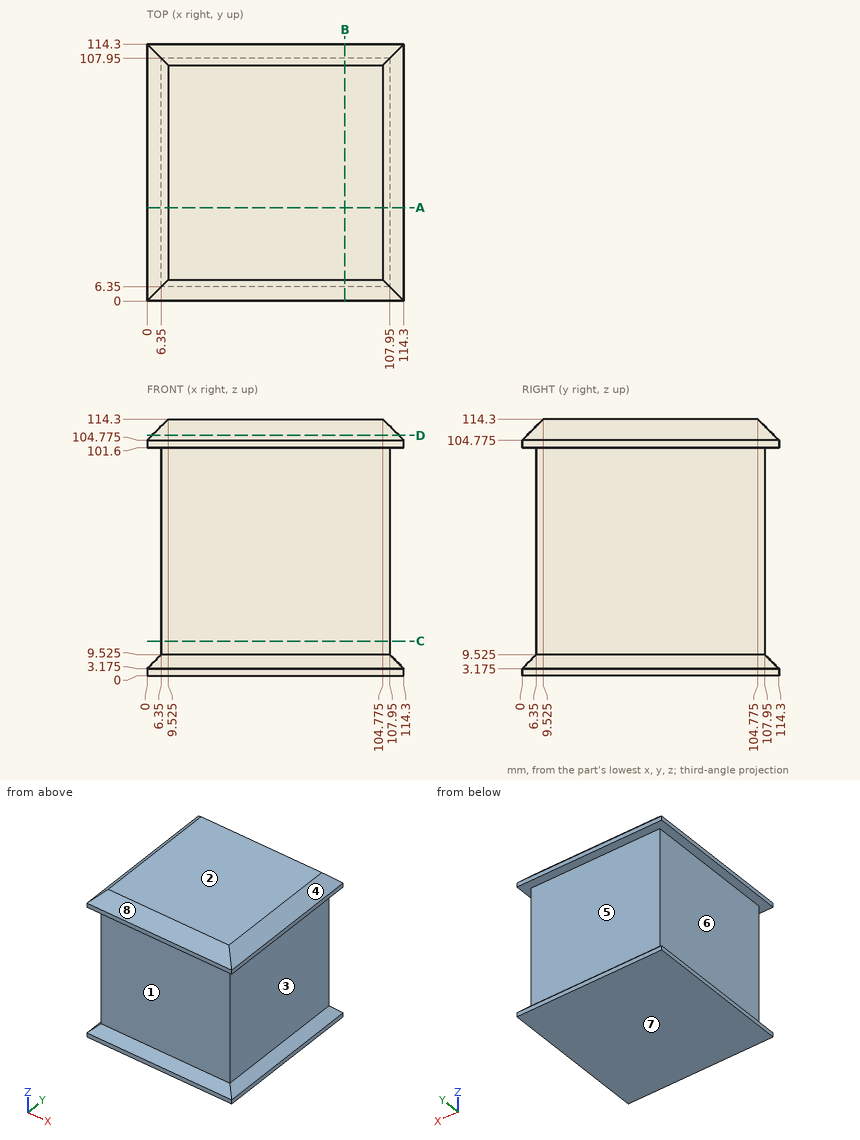
Design review of the part shown in the three views and the two pictorial views. Dimensions are in mm from the part's minimum x, y and z. A direction names the side the tool comes from. Round coordinates to 2 decimals unless told otherwise and drop trailing zeros. Write each loop counter-clockwise with the first axis right and the second up, starting at its lowest first coordinate (ties: lowest second). Pieces come first, ordered by that corner, then holes. Notation, with made-up numbers: (17, -30) - (68, -30) arc R32 cw to (68, 4) - close; hole circle Ø2 at (49.5, 53). An arc over 180 degrees is marked (long way). Answer as CSV lines item,"result". Start each with the question number.
(1) Add section C-C, the plane z = 15.5. State the section outline as (x, y) points, plus the area to 3 significant figures.
(2) Add section D-D, the plane z = 107. State the section outline as (x, y) points (3 decimals).
(3) For line 1 (Y direction, x = 36, z = 85); line 2 (Z direction, x = 5, y = 74) (3 decimals), list the stretches that pass through material, from the lowest coordinate up.
(4) Mouldability with a two-part tool opening along Z and no side actions: class the marked faces 6, 7 and 8 as +Z half, -Z half, draft (parallel to the pull), parting line (faces both ways), or undercut.
(5) For pin 1 (4 mm diameter, centred on x = 100.5, z = 64, fed in from +Y); pin 2 (3 mm diameter, centred on x = 39, y = 98.5, fed in from -Z); pin 3 (5 mm diameter, centred on y = 15.5, z = 93.5, fed in from -X); pin 4 (4 mm diameter, centred on y = 51, z = 95.5, fed in from +X), all flat-tipped, find the tip position at first contact; note any pin that passes through.
(6) Add section A-A, the plane y = 41.5. State the section outline as (x, z) points (3 decimals), plus the area to 3 significant figures.
(7) Machinability: for the marked faces 1, 2, 3, 4 and 5, which of the approach directions +Z, -Z, +X, -X, +Y, -Y give a long, thin tool a straight path to every point of the face, cutting with its end or side? Answer none if there is none.
From the geometry:
1,outline,"(6.35, 6.35) - (107.95, 6.35) - (107.95, 107.95) - (6.35, 107.95) - close"
1,area,"10,300 mm²"
2,outline,"(2.225, 2.225) - (112.075, 2.225) - (112.075, 112.075) - (2.225, 112.075) - close"
3,line 1,"y = 6.35 to 107.95"
3,line 2,"z = 0 to 8.175, 101.6 to 109.775"
4,face 6,"undercut"
4,face 7,"-Z half"
4,face 8,"+Z half"
5,pin 1,"stops at y = 107.95"
5,pin 2,"stops at z = 0"
5,pin 3,"stops at x = 6.35"
5,pin 4,"stops at x = 107.95"
6,outline,"(0, 0) - (114.3, 0) - (114.3, 3.175) - (107.95, 9.525) - (107.95, 101.6) - (114.3, 101.6) - (114.3, 104.775) - (104.775, 114.3) - (9.525, 114.3) - (0, 104.775) - (0, 101.6) - (6.35, 101.6) - (6.35, 9.525) - (0, 3.175) - close"
6,area,"11,800 mm²"
7,face 1,"+X, -X, -Y"
7,face 2,"+Z, +X, -X, +Y, -Y"
7,face 3,"+X, +Y, -Y"
7,face 4,"+Z, +X, +Y, -Y"
7,face 5,"+X, -X, +Y"
